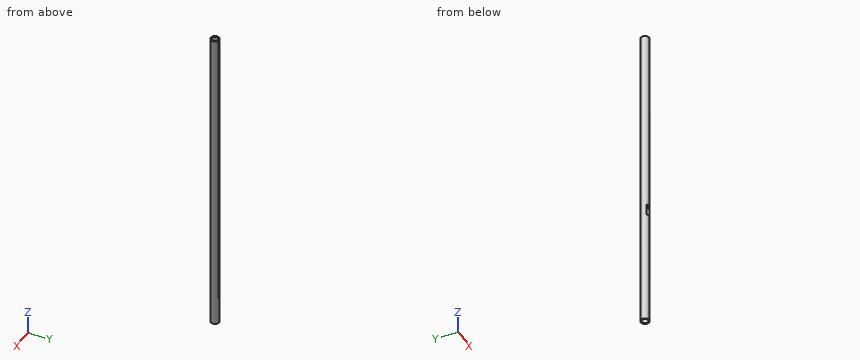
```python
from build123d import *

# Parameters (mm, degrees)
SKETCH1_R           = 0.735
SKETCH1_R_2         = 0.535
BOSS_EXTRUDE1_DEPTH = 57
SKETCH2_W           = 0.45
SKETCH2_H           = 53
CUT_EXTRUDE1_DEPTH  = 1.735
SKETCH3_W           = 1
SKETCH3_H           = 2
CUT_EXTRUDE2_DEPTH  = 1.735


with BuildPart() as part:
    # Sketch1 → Boss-Extrude1 (new body)
    with BuildSketch(Plane.XY):
        Circle(SKETCH1_R)
        Circle(SKETCH1_R_2, mode=Mode.SUBTRACT)
    extrude(amount=BOSS_EXTRUDE1_DEPTH)

    # Sketch2 → Cut-Extrude1 (cut, through all)
    with BuildSketch(Plane(origin=(0, 0, 0), x_dir=(1, 0, 0), z_dir=(0, 1, 0))):
        with Locations((0, -31.5)):
            Rectangle(SKETCH2_W, SKETCH2_H)
    extrude(amount=CUT_EXTRUDE1_DEPTH, mode=Mode.SUBTRACT)

    # Sketch3 → Cut-Extrude2 (cut, through all)
    with BuildSketch(Plane(origin=(0, 0, 0), x_dir=(1, 0, 0), z_dir=(0, 1, 0))):
        with Locations((0, -22)):
            Rectangle(SKETCH3_W, SKETCH3_H)
    extrude(amount=-CUT_EXTRUDE2_DEPTH, mode=Mode.SUBTRACT)


solid = part.part
```
The listing builds one solid part. Answer for the finished solid, in the listing's coordinates (mm). Round coordinates to 2 decimals unless told otherwise and drop trailing zeros. Order: outer loops, then holes, each group sorted by start corner. A loop starts at its lowest first (then second) coordinate and runs counter-clockwise, first axis right, second up. Notation, with made-up numbers: (-12.75, 27) -> (3.25, 27) arc R31 ccw to (3.25, 53) -> close; hole circle Ø7 at (28.5, -12). An arc over 180 degrees is marked (long way). Answer as CSV lines item,"result".
Q1. A cutting plane is placed at B-B on z = 9. Determine the outline of the cut face in (x, y) (3 decimals).
Computed values:
outline,"(-0.225, 0.485) -> (-0.225, 0.7) arc R0.735 ccw (long way) to (0.225, 0.7) -> (0.225, 0.485) arc R0.535 cw (long way) to start"
Q2. A cutting plane is placed at A-A on x = 0. Determine the outline of the cut face in (y, z) (3 decimals).
Computed values:
outline,"(-0.735, 0) -> (-0.535, 0) -> (-0.535, 21) -> (-0.735, 21) -> close; (-0.735, 23) -> (-0.535, 23) -> (-0.535, 57) -> (-0.735, 57) -> close; (0.535, 0) -> (0.735, 0) -> (0.735, 5) -> (0.535, 5) -> close"
Q3. Consider line 1 (X direction, y = 0, z = 45.5) (3 decimals); line 2 (X direction, y = 0.5, z = 38.5) (3 decimals); line 3 (Y direction, x = 0, z = 41) (3 decimals). Determine where each line is inside the solid, lowest interval first. Write a range as from..to.
Computed values:
line 1,"x = -0.735..-0.535, 0.535..0.735"
line 2,"x = -0.539..-0.225, 0.225..0.539"
line 3,"y = -0.735..-0.535"
